Work out the finished part from the listing and answer in its coordinate system (mm). A direction names the side the tool comes from. Coordinates: 2 decimals unless noted, no trailing zeros. Order: outer loops, then holes, each group sorted by start corner. A loop starts at its lowest first (then second) coordinate and runs counter-clockwise, first axis right, second up. Notation, with made-up numbers: M 26.25,-32.75 L 85.25,-32.75 A28 cw 85.25,0.25 Z; hole C -28,14 d1. An arc over 180 degrees is marked long. Answer in a Markdown table with one row per item. Add a question column.
Item 1: Which of the six approach directions +Z, -Z, +X, -X, +Y, -Y give full straight-line access (tool end or side, diameter ignored) to faces 1 (the face through (-309, 14, 97.86)), 2 (the face through (-310, 34, 77.86)), 3 (the face through (-281.56, 51.5, 116.13))?
Item 2: The part is cut by section C-C (x = -347). Write down the section's boundary in (y, z), then the cut area to 3 significant figures.
Item 3: Flat-ended cylindrical pins translate along their axes: pin 1 Ø9 at (x, z) = (-334.43, 114.86) entering from -Y; pin 2 Ø5 at (x, z) = (-284, 112) entering from +Y; pin 3 Ø3 at (y, z) = (26.5, 69) entering from +X; pin 4 Ø5 at (x, y) = (-349.31, 42) entering from -Z. Find the tip coordinate at first contact, or state that the pin passes through.
Item 4: The part is cut by section D-D (y = 35). Write down the section's boundary in (x, z).
Item 5: The part is cut by section A-A (z = 123.5). Write down the section's boundary in (x, y).
Item 6: The part is cut by section B-B (y = 42). Write down the section's boundary in (x, z), then the cut area to 3 significant figures.
Item 7: The mould has two halves that part along X. Classify faces 4 (the face through (-308.614, 54.145, 126.958)), 5 (the face through (-358.459, 54.098, 102.51)), 6 (the face through (-331.685, 40.646, 114.74)): released by +X, released by -X, zero draft, split by the parting line, or undercut.
Item 8: Consider line 1 (X direction, y = 44, z = 123.5); line 2 (Y direction, x = -311, z = 124); line 3 (Z direction, x = -307.5, y = 17). Determine where each line is inside the solid, lowest interval first. Write a range as from..to.
from build123d import *

# Parameters (mm, degrees)
ESBO_O1_W                                            = 100
ESBO_O1_H                                            = 40
ESBO_O1_R                                            = 4
RESSALTO_EXTRUS_O1_DEPTH                             = 50
FILETE1_R                                            = 3
ESBO_O3_W                                            = 30.13686718
ESBO_O3_H                                            = 15.092425978
CORTE_EXTRUS_O1_DEPTH                                = 1
CORTE_EXTRUS_O1_DEPTH_BACK                           = 101
ESBO_O4_R                                            = 17.5
RESSALTO_EXTRUS_O2_DEPTH                             = 20
RESSALTO_EXTRUS_O2_DEPTH_BACK                        = 20
REBAIXO_PARA_PARAFUSO_DE_CABE_A_SEXTAVAD_D           = 5.5
REBAIXO_PARA_PARAFUSO_DE_CABE_A_SEXTAVAD_CBORE_D     = 12.238
REBAIXO_PARA_PARAFUSO_DE_CABE_A_SEXTAVAD_CBORE_DEPTH = 3.5


with BuildPart() as part:
    # Esboço1 → Ressalto-extrusão1 (new body)
    with BuildSketch(Plane.XY.offset(127.860451464)):
        with Locations((-309.31398478, 35)):
            Rectangle(ESBO_O1_W, ESBO_O1_H)
        with Locations((-349.31398478, 42)):
            Circle(ESBO_O1_R, mode=Mode.SUBTRACT)
        with Locations((-269.31398478, 42)):
            Circle(ESBO_O1_R, mode=Mode.SUBTRACT)
    extrude(amount=-RESSALTO_EXTRUS_O1_DEPTH)

    # Filete1
    filete1_edges = [part.edges().sort_by_distance(p)[0] for p in [
        (-309.31398478, 55, 77.860451464),
        (-309.31398478, 55, 127.860451464),
        (-359.31398478, 55, 102.860451464),
        (-259.31398478, 55, 102.860451464),
    ]]
    fillet(filete1_edges, radius=FILETE1_R)

    # Esboço3 → Corte-extrusão1 (cut, two sides)
    with BuildSketch(Plane.ZY.offset(359.31398478)) as corte_extrus_o1_sk:
        with Locations((112.792017874, 22.546212989)):
            Rectangle(ESBO_O3_W, ESBO_O3_H)
    extrude(amount=CORTE_EXTRUS_O1_DEPTH, mode=Mode.SUBTRACT)
    extrude(corte_extrus_o1_sk.sketch, amount=-CORTE_EXTRUS_O1_DEPTH_BACK, mode=Mode.SUBTRACT)

    # Esboço4 → Ressalto-extrusão2 (add, two sides)
    with BuildSketch(Plane(origin=(0, 0, 77.860451464), x_dir=(-1, 0, 0), z_dir=(0, 0, -1))) as ressalto_extrus_o2_sk:
        with Locations((309.31398478, 14.975825016)):
            Circle(ESBO_O4_R)
    extrude(amount=RESSALTO_EXTRUS_O2_DEPTH)
    extrude(ressalto_extrus_o2_sk.sketch, amount=-RESSALTO_EXTRUS_O2_DEPTH_BACK)

    # Rebaixo para parafuso de cabeça sextavada de M51 (through all)
    with Locations(Plane(origin=(0, 55, 0), x_dir=(1, 0, 0), z_dir=(0, 1, 0))):
        with Locations((-284.195309224, -114.860451464), (-334.432660336, -114.860451464), (-309.31398478, -107.896538756)):
            CounterBoreHole(REBAIXO_PARA_PARAFUSO_DE_CABE_A_SEXTAVAD_D / 2, REBAIXO_PARA_PARAFUSO_DE_CABE_A_SEXTAVAD_CBORE_D / 2, REBAIXO_PARA_PARAFUSO_DE_CABE_A_SEXTAVAD_CBORE_DEPTH)


solid = part.part
Reply:
| question | item | result |
|---|---|---|
| 1 | face 1 | +Z, +X, -X, -Y |
| 1 | face 2 | -Z, +Y |
| 1 | face 3 | +Y |
| 2 | outline | M 15,77.86 L 38.74,77.86 L 38.74,127.86 L 30.09,127.86 L 30.09,97.72 L 15,97.72 Z; M 45.26,77.86 L 52,77.86 A3 ccw 55,80.86 L 55,124.86 A3 ccw 52,127.86 L 45.26,127.86 Z |
| 2 | area | 1,220 mm2 |
| 3 | pin 1 | stops at y = 30.09 |
| 3 | pin 2 | stops at y = 51.5 |
| 3 | pin 3 | stops at x = -294.97 |
| 3 | pin 4 | passes through |
| 4 | outline | M -359.31,77.86 L -259.31,77.86 L -259.31,127.86 L -359.31,127.86 Z; hole C -334.43,114.86 d5.5; hole C -309.31,107.9 d5.5; hole C -284.2,114.86 d5.5 |
| 5 | outline | M -359.31,30.09 L -259.31,30.09 L -259.31,52 A3 ccw -262.31,55 L -356.31,55 A3 ccw -359.31,52 Z; hole C -349.31,42 d8; hole C -269.31,42 d8 |
| 6 | outline | M -359.31,77.86 L -353.31,77.86 L -353.31,127.86 L -359.31,127.86 Z; M -345.31,77.86 L -273.31,77.86 L -273.31,127.86 L -345.31,127.86 Z; M -265.31,77.86 L -259.31,77.86 L -259.31,127.86 L -265.31,127.86 Z; hole C -334.43,114.86 d5.5; hole C -309.31,107.9 d5.5; hole C -284.2,114.86 d5.5 |
| 6 | area | 4,130 mm2 |
| 7 | face 4 | zero draft |
| 7 | face 5 | released by -X |
| 7 | face 6 | undercut |
| 8 | line 1 | x = -359.31..-352.78, -345.85..-272.78, -265.85..-259.31 |
| 8 | line 2 | y = 30.09..55 |
| 8 | line 3 | z = 57.86..97.86 |
